from build123d import *

# Parameters (mm, degrees)
F0_R     = 34.5257671678
F1_DEPTH = 25
F2_SIZE2 = 10
F2_SIZE  = 20
F4_DEPTH = 25


with BuildPart() as f1:
    # F0 (on Top) → F1 (new body)
    with BuildSketch(Plane.XY):
        Circle(F0_R)
    extrude(amount=F1_DEPTH)

    # F2
    f2_edges = [f1.edges().sort_by_distance(p)[0] for p in [
        (-34.525767, 0, 25),
    ]]
    f2_side = f1.faces().sort_by_distance((0, 0, 25))[0]
    chamfer(f2_edges, length=F2_SIZE, length2=F2_SIZE2, reference=f2_side)

    # F3 (on face) → F4 (cut)
    with BuildSketch(Plane.XY.offset(25)):
        with BuildLine():
            Line((-3.6215493205, -34.3353022273), (-3.6215493205, -14.0670640978))
            ThreePointArc((-3.6215493205, -14.0670640978), (-8.899217089, 11.4804985525), (14.5257671678, 0))
            ThreePointArc((14.5257671678, 0), (11.4804985525, -8.899217089), (3.6215493205, -14.0670640978))
            Line((3.6215493205, -14.0670640978), (3.6215493205, -34.3353022273))
            ThreePointArc((3.6215493205, -34.3353022273), (25.6618916601, -23.0975304946), (34.5257671678, 0))
            ThreePointArc((34.5257671678, 0), (-23.0975304946, 25.6618916601), (-3.6215493205, -34.3353022273))
        make_face()
    extrude(amount=-F4_DEPTH, mode=Mode.SUBTRACT)


solid = f1.part
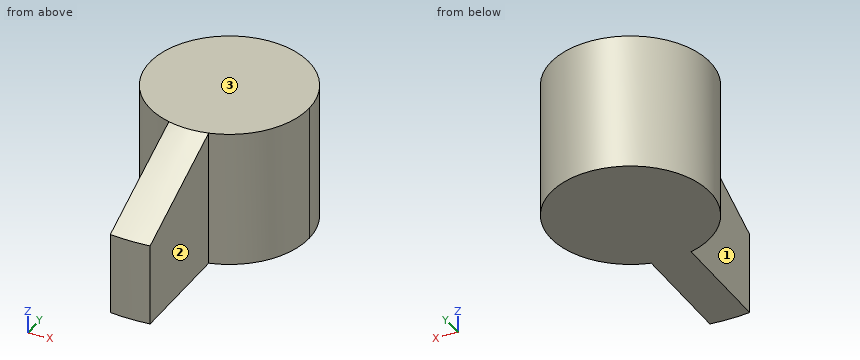
Read the model definition and answer for the solid it produces. Units are mm, in the model's axes. Face numbers are marked on the shaded views. A direction names the side the tool comes from. Round coordinates to 2 decimals unless told otherwise and drop trailing zeros. Write each loop counter-clockwise with the first axis right and the second up, starting at its lowest first coordinate (ties: lowest second). Pieces come first, ordered by that corner, then holes. Notation, with made-up numbers: M 86.5,19.25 L 140.5,19.25 A10 cw 140.5,35.25 Z; hole C 82.25,8 d5. An arc over 180 degrees is marked long. Use a Markdown table: item, result.
1) Straight lines are drawn through the part: line 1 along X through (y, z) = (-17, 7); line 2 along Y through (x, z) = (0.75, 14); line 3 along Y through (x, z) = (-10, 21). For each, find the intervals that lie inside material, in ascending order. Write a range as [from, to].
Answers follow:
| item | result |
|---|---|
| line 1 | x = [-3.62, 3.62] |
| line 2 | y = [-34.52, 14.51] |
| line 3 | y = [-10.54, 10.54] |
2) A tool of negligible diameter and unlimited length cuts with its end or side. For the marked faces 1, 2 and 3, from which of +Z, -Z, +X, -X, +Y, -Y can it reach the whole face along a straight path? Write none if from no direction.
Answers follow:
| item | result |
|---|---|
| face 1 | +Z, -Z, -X, -Y |
| face 2 | +Z, -Z, +X, -Y |
| face 3 | +Z, +X, -X, +Y, -Y |
3) The part is cut by section B-B (z = 14). Write down the section's boundary in (x, y), plus the area to 3 significant figures.
Answers follow:
| item | result |
|---|---|
| outline | M -3.62,-34.34 A34.53 ccw 3.62,-34.34 L 3.62,-14.07 A14.53 ccw long -3.62,-14.07 Z |
| area | 808 mm2 |
4) Flat-ended cylindrical pins translate along their axes: pin 1 (5 mm diameter, centred on x = 1, y = -21, fed in from +Z); pin 2 (1.5 mm diameter, centred on x = -0.5, y = -21.5, fed in from +Z) (3 decimals); pin 3 (12 mm diameter, centred on x = -10, z = 21, fed in from +Y). Find the tip coordinate at first contact, or state that the pin passes through.
Answers follow:
| item | result |
|---|---|
| pin 1 | stops at z = 23 |
| pin 2 | stops at z = 21.885 |
| pin 3 | stops at y = 13.96 |
5) The part is cut by section C-C (x = 6.5). Write down the section's boundary in (y, z).
Answers follow:
| item | result |
|---|---|
| outline | M -12.99,0 L 12.99,0 L 12.99,25 L -12.99,25 Z |
6) The part is cut by section A-A (x = 0). Write down the section's boundary in (y, z), plus the area to 3 significant figures.
Answers follow:
| item | result |
|---|---|
| outline | M -34.53,0 L 14.53,0 L 14.53,25 L -14.53,25 L -34.53,15 Z |
| area | 1,130 mm2 |
